Verification items for the finished model (mm, model axes). Coordinates: 2 decimals unless noted, no trailing zeros. Order: outer loops, then holes, each group sorted by start corner. A loop starts at its lowest first (then second) coordinate and runs counter-clockwise, first axis right, second up. Notation, with made-up numbers: (35, -24.5) -> (61, -24.5) arc R21 ccw to (61, 2.5) -> close; hole circle Ø1 at (-15.75, 2.25). An arc over 180 degrees is marked (long way). Write item = value, one per line. Start each with the question number.
1. Cross-section at B-B on z = 10. Record the cut outline in (x, y) (3 decimals).
2. Cross-section at D-D on z = -11. Record the cut outline in (x, y) (3 decimals), plus the area to 3 significant figures.
3. Go/stop test with flat-tipped pins: P1, Ø1.7, axis at x = -48.5, y = 0.5, coming from the -Z side (3 decimals); P2, Ø1.5, axis at y = 0, z = 10.5, coming from the +X side; P3, Ø1.5, axis at x = -70.5, y = 2.5, coming from the -Z side; P4, Ø3, axis at x = -21, y = 2.5, coming from the +Z side. Record where each tip stops, or that it passes through.
4. Thickness scan on line 1 along Z through (x, y) = (-11.5, 2.45) (3 decimals); line 2 along Z through (x, y) = (-15.5, -0.1) (3 decimals); line 3 along Z through (x, y) = (18, 0.35). Record the ranges inside material, lowest first. Write a range as from..to.
5. Cross-section at A-A on y = 1.2. Record the cut outline in (x, z) (3 decimals).
6. Cross-section at C-C on x = 72. Record the cut outline in (y, z) (3 decimals).
from build123d import *

# Parameters (mm, degrees)
F2_DEPTH = 1.905
F3_DEPTH = 3.81
F4_W     = 69.85
F4_H     = 5.08
F5_DEPTH = 5.716


with BuildPart() as f2:
    # F0 (on Front) → F2 (new body)
    with BuildSketch(Plane.XZ):
        with BuildLine():
            Line((-76.2, 15.875), (-76.2, 0))
            Line((-76.2, 0), (-60.325, 0))
            ThreePointArc((-60.325, 0), (-64.9746798487, 11.2253201513), (-76.2, 15.875))
        make_face()
        with BuildLine():
            Line((-60.325, 0), (-76.2, 0))
            Line((-76.2, 0), (-76.2, -15.875))
            ThreePointArc((-76.2, -15.875), (-64.9746798487, -11.2253201513), (-60.325, 0))
        make_face()
        with BuildLine():
            Line((-76.2, -15.875), (-76.2, 0))
            Line((-76.2, 0), (-76.2, 15.875))
            ThreePointArc((-76.2, 15.875), (-92.075, 0), (-76.2, -15.875))
        make_face()
        with BuildLine():
            ThreePointArc((-76.2, 15.875), (-64.9746798487, 11.2253201513), (-60.325, 0))
            Line((-60.325, 0), (60.325, 0))
            ThreePointArc((60.325, 0), (64.9746798487, 11.2253201513), (76.2, 15.875))
            Line((76.2, 15.875), (-76.2, 15.875))
        make_face()
        with BuildLine():
            Line((60.325, 0), (-60.325, 0))
            ThreePointArc((-60.325, 0), (-64.9746798487, -11.2253201513), (-76.2, -15.875))
            Line((-76.2, -15.875), (76.2, -15.875))
            ThreePointArc((76.2, -15.875), (64.9746798487, -11.2253201513), (60.325, 0))
        make_face()
        with BuildLine():
            ThreePointArc((76.2, 15.875), (64.9746798487, 11.2253201513), (60.325, 0))
            Line((60.325, 0), (76.2, 0))
            Line((76.2, 0), (76.2, 15.875))
        make_face()
        with BuildLine():
            Line((76.2, 0), (60.325, 0))
            ThreePointArc((60.325, 0), (64.9746798487, -11.2253201513), (76.2, -15.875))
            Line((76.2, -15.875), (76.2, 0))
        make_face()
        with BuildLine():
            Line((76.2, 0), (76.2, -15.875))
            ThreePointArc((76.2, -15.875), (87.4253201513, -11.2253201513), (92.075, 0))
            ThreePointArc((92.075, 0), (87.4253201513, 11.2253201513), (76.2, 15.875))
            Line((76.2, 15.875), (76.2, 0))
        make_face()
    extrude(amount=F2_DEPTH)

    # F1 (on Front) → F3 (join)
    with BuildSketch(Plane.XZ):
        with BuildLine():
            ThreePointArc((76.2, -13.97), (62.23, 0), (76.2, 13.97))
            Line((76.2, 13.97), (-76.2, 13.97))
            ThreePointArc((-76.2, 13.97), (-66.3217182668, 9.8782817332), (-62.23, 0))
            ThreePointArc((-62.23, 0), (-66.3217182668, -9.8782817332), (-76.2, -13.97))
            Line((-76.2, -13.97), (76.2, -13.97))
        make_face()
        with BuildLine():
            ThreePointArc((90.17, 0), (86.0782817332, 9.8782817332), (76.2, 13.97))
            Line((76.2, 13.97), (76.2, -13.97))
            ThreePointArc((76.2, -13.97), (86.0782817332, -9.8782817332), (90.17, 0))
        make_face()
        with BuildLine():
            Line((76.2, -13.97), (76.2, 13.97))
            ThreePointArc((76.2, 13.97), (62.23, 0), (76.2, -13.97))
        make_face()
        with BuildLine():
            ThreePointArc((-62.23, 0), (-66.3217182668, 9.8782817332), (-76.2, 13.97))
            Line((-76.2, 13.97), (-76.2, -13.97))
            ThreePointArc((-76.2, -13.97), (-66.3217182668, -9.8782817332), (-62.23, 0))
        make_face()
        with BuildLine():
            Line((-76.2, -13.97), (-76.2, 13.97))
            ThreePointArc((-76.2, 13.97), (-90.17, 0), (-76.2, -13.97))
        make_face()
    extrude(amount=-F3_DEPTH)

    # F4 (on face) → F5 (cut, through all)
    with BuildSketch(Plane.XZ.offset(1.905)):
        with Locations((-38.1, 10.795)):
            Rectangle(F4_W, F4_H)
    extrude(amount=-F5_DEPTH, mode=Mode.SUBTRACT)


solid = f2.part
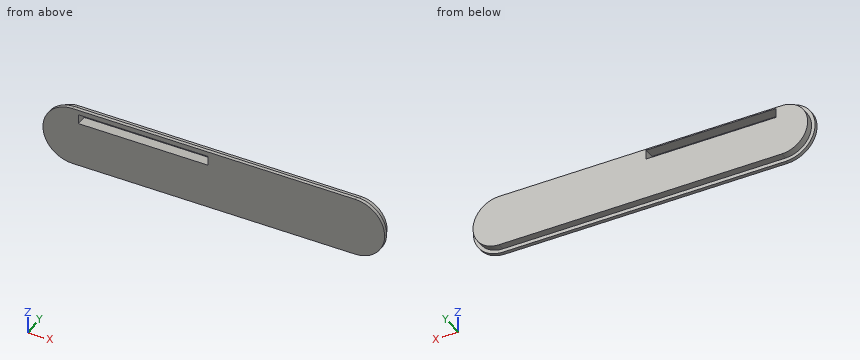
Worked out:
q1.outline = (-88.529, -1.905) -> (-73.025, -1.905) -> (-73.025, 3.81) -> (-85.955, 3.81) -> (-85.955, 0) -> (-88.529, 0) -> close; (-3.175, -1.905) -> (88.529, -1.905) -> (88.529, 0) -> (85.955, 0) -> (85.955, 3.81) -> (-3.175, 3.81) -> close
q2.outline = (-87.646, -1.905) -> (87.646, -1.905) -> (87.646, 0) -> (84.812, 0) -> (84.812, 3.81) -> (-84.812, 3.81) -> (-84.812, 0) -> (-87.646, 0) -> close
q2.area = 980 mm²
q3.P1 = -15.875
q3.P2 = 88.73
q3.P3 = -13.97
q3.P4 = 13.97
q4.line_1 = -13.97..8.255, 13.335..13.97
q4.line_2 = -15.875..8.255, 13.335..15.875
q4.line_3 = -13.97..13.97
q5.outline = (-76.2, -13.97) -> (76.2, -13.97) arc R13.97 ccw to (76.2, 13.97) -> (-76.2, 13.97) arc R13.97 ccw to start; hole (-73.025, 8.255) -> (-3.175, 8.255) -> (-3.175, 13.335) -> (-73.025, 13.335) -> close
q6.outline = (-1.905, -15.875) -> (0, -15.875) -> (0, -13.97) -> (3.81, -13.97) -> (3.81, 13.97) -> (0, 13.97) -> (0, 15.875) -> (-1.905, 15.875) -> close
